Check sheet for the modelled part. Datum: model origin and axes. Units: mm. Round coordinates to 2 decimals unless told otherwise and drop trailing zeros. Loops run counter-clockwise (first coordinate to the right, second up) from the corner with the lowest first, then second, coordinate; pieces in that order, holes last. Notation, with made-up numbers: (59, 88.25) - (111, 88.25) arc R13 ccw to (111, 111.25) - close; hole circle Ø5 at (2.25, 76). An arc over 180 degrees is marked (long way). Put each result on its own line as item: value. Start each with the question number.
Item 1: Gauge pin test, flat ends, axial feed: pin 1 Ø1 at (x, z) = (0, 1) entering from +Y (3 decimals); pin 2 Ø0.9 at (x, z) = (-36, 0) entering from -Y (3 decimals); pin 3 Ø1.6 at (x, z) = (39, 0) entering from +Y. Record the tip position at first contact, or that the pin passes through.
Item 2: Section check A-A, the plane x = -12. Record the cut outline in (y, z) (1 decimal), and give its area (3 significant figures).
Item 3: Material ranges on line 1 along X through (y, z) = (2.5, 0.9) (3 decimals); line 2 along Y through (x, z) = (13.5, 1.2) (3 decimals), recorded low to high.
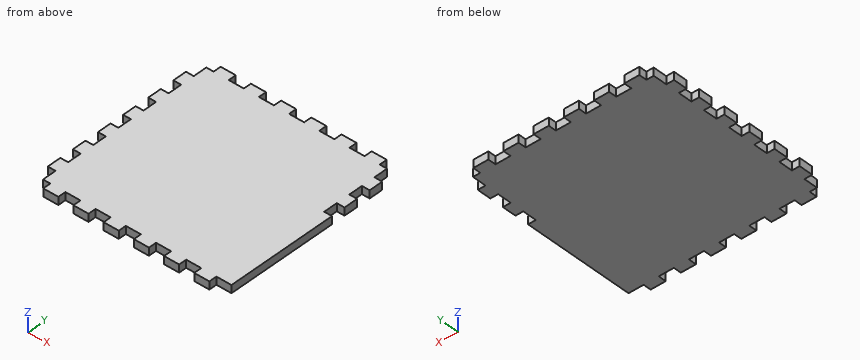
from build123d import *

# Parameters (mm, degrees)
SKETCH1_W           = 80
SKETCH1_H           = 80
BOSS_EXTRUDE1_DEPTH = 1.5875
SKETCH3_OUTSIDE_W   = 104.636
SKETCH3_OUTSIDE_H   = 104.636
CUT_EXTRUDE2_DEPTH  = 57.657573413
SKETCH4_W           = 3.175
SKETCH4_H           = 45.323076923
BOSS_EXTRUDE2_DEPTH = 3.175


with BuildPart() as part:
    # Sketch1 → Boss-Extrude1 (new, symmetric)
    with BuildSketch(Plane.XY):
        Rectangle(SKETCH1_W, SKETCH1_H)
    extrude(amount=BOSS_EXTRUDE1_DEPTH, both=True)

    # Sketch3 outside → Cut-Extrude2 (cut, through all)
    with BuildSketch(Plane.XY.offset(1.5875)):
        Rectangle(SKETCH3_OUTSIDE_W, SKETCH3_OUTSIDE_H)
        Polygon((-36.825, 36.825), (-33.846153846, 36.825), (-33.846153846, 40), (-27.692307692, 40), (-27.692307692, 36.825), (-21.538461538, 36.825), (-21.538461538, 40), (-15.384615385, 40), (-15.384615385, 36.825), (-9.230769231, 36.825), (-9.230769231, 40), (-3.076923077, 40), (-3.076923077, 36.825), (3.076923077, 36.825), (3.076923077, 40), (9.230769231, 40), (9.230769231, 36.825), (15.384615385, 36.825), (15.384615385, 40), (21.538461538, 40), (21.538461538, 36.825), (27.692307692, 36.825), (27.692307692, 40), (33.846153846, 40), (33.846153846, 36.825), (36.825, 36.825), (36.825, 31.159615385), (40, 31.159615385), (40, 25.494230769), (36.825, 25.494230769), (36.825, 19.828846154), (40, 19.828846154), (40, 14.163461538), (36.825, 14.163461538), (36.825, 8.498076923), (40, 8.498076923), (40, 2.832692308), (36.825, 2.832692308), (36.825, -2.832692308), (40, -2.832692308), (40, -8.498076923), (36.825, -8.498076923), (36.825, -14.163461538), (40, -14.163461538), (40, -19.828846154), (36.825, -19.828846154), (36.825, -25.494230769), (40, -25.494230769), (40, -31.159615385), (36.825, -31.159615385), (36.825, -36.825), (33.846153846, -36.825), (33.846153846, -40), (27.692307692, -40), (27.692307692, -36.825), (21.538461538, -36.825), (21.538461538, -40), (15.384615385, -40), (15.384615385, -36.825), (9.230769231, -36.825), (9.230769231, -40), (3.076923077, -40), (3.076923077, -36.825), (-3.076923077, -36.825), (-3.076923077, -40), (-9.230769231, -40), (-9.230769231, -36.825), (-15.384615385, -36.825), (-15.384615385, -40), (-21.538461538, -40), (-21.538461538, -36.825), (-27.692307692, -36.825), (-27.692307692, -40), (-33.846153846, -40), (-33.846153846, -36.825), (-36.825, -36.825), (-36.825, -31.159615385), (-40, -31.159615385), (-40, -25.494230769), (-36.825, -25.494230769), (-36.825, -19.828846154), (-40, -19.828846154), (-40, -14.163461538), (-36.825, -14.163461538), (-36.825, -8.498076923), (-40, -8.498076923), (-40, -2.832692308), (-36.825, -2.832692308), (-36.825, 2.832692308), (-40, 2.832692308), (-40, 8.498076923), (-36.825, 8.498076923), (-36.825, 14.163461538), (-40, 14.163461538), (-40, 19.828846154), (-36.825, 19.828846154), (-36.825, 25.494230769), (-40, 25.494230769), (-40, 31.159615385), (-36.825, 31.159615385), align=None, mode=Mode.SUBTRACT)
    extrude(amount=-CUT_EXTRUDE2_DEPTH, mode=Mode.SUBTRACT)

    # Sketch4 → Boss-Extrude2 (add)
    with BuildSketch(Plane.XY.offset(1.5875)):
        with Locations((38.4125, -14.163461539)):
            Rectangle(SKETCH4_W, SKETCH4_H)
    extrude(amount=-BOSS_EXTRUDE2_DEPTH)


solid = part.part
Check result:
1. pin 1: y = 36.825
1. pin 2: y = -36.825
1. pin 3: y = 31.16
2. outline: (-36.8, -1.6) - (36.8, -1.6) - (36.8, 1.6) - (-36.8, 1.6) - close
2. area: 234 mm²
3. line 1: -36.825 to 40
3. line 2: -36.825 to 36.825
